CAD build for the part. Positions are in the model's coordinates, mm. A direction names the side the tool comes from. Coordinates: 2 decimals unless noted, no trailing zeros. Loops run counter-clockwise (first coordinate to the right, second up) from the corner with the lowest first, then second, coordinate; pieces in that order, holes last.
1) Two-plate mould, pull along X, no slides. Class faces 1 (the flat face through (-20, 3, -15)), 2 (the flat face through (-33.8, 5, -23)), 3 (the flat face through (-53, 3, -10)): +X half, -X half, draft (parallel to the pull), parting line (faces both ways), or undercut.
2) Pin check, flat tips, straight feed: pin 1 Ø3.5 at (x, z) = (-24.5, -27) entering from +Y; pin 2 Ø1 at (y, z) = (5, -1.5) entering from +X; pin 3 Ø5.5 at (x, z) = (-82.5, -6) entering from +Y; pin 4 Ø4 at (x, z) = (-81.5, -4.5) entering from -Y. Stop position of each tip, or through.
3) Saw through at A-A, the plane x = -59.5. Write the cut outline in (y, z), and give its area (3 significant figures).
4) Wall check: line 1 along X through (y, z) = (3.5, -13); line 2 along Z through (x, y) = (-41, 1.5); line 3 along X through (y, z) = (2.5, -6). Give the ranges that are in metal, low to high.
5) Saw through at D-D, the plane y = 5.75. Write the cut outline in (x, z).
6) Saw through at B-B, the plane z = -14.5. Write the cut outline in (x, y).
7) Saw through at C-C, the plane x = -82.5. Write the cut outline in (y, z), and give its area (3 significant figures).
8) Which spindle directions (+Z, -Z, +X, -X, +Y, -Y) get a long thin tool onto all of the face, cutting with end or side? Do faces 4 (the flat face through (-85.1, 4, -23.9)), 5 (the cylindrical face through (-38.4, 3.45, -10.57)), 6 (the flat face through (-27.8, 5, -1)). Say none if no direction does.
```python
from build123d import *

# Parameters (mm, degrees)
SKETCH_1_W           = 88
SKETCH_1_H           = 30
EXTRUDE_1_DEPTH      = 3
SKETCH_2_W           = 27.8
SKETCH_2_H           = 30
CUT_EXTRUDE_1_DEPTH  = 1
SKETCH_3_R           = 1.45
CUT_EXTRUDE_2_DEPTH  = 11
SKETCH_4_R           = 2.45
CUT_EXTRUDE_4_DEPTH  = 11
SKETCH_5_W           = 30.2
SKETCH_5_H           = 10
CUT_EXTRUDE_5_DEPTH  = 11
FILLET_1_R           = 2
SKETCH_6_W           = 5
SKETCH_6_H           = 30
CUT_EXTRUDE_6_DEPTH  = 10
SKETCH_9_W           = 60.2
SKETCH_9_H           = 30
SKETCH_9_R           = 2.45
EXTRUDE_4_DEPTH      = 4
EXTRUDE_START        = 1
SKETCH_7_W           = 22.8
SKETCH_7_H           = 30
SKETCH_7_R           = 1.45
EXTRUDE_5_DEPTH      = 1
SKETCH_11_W          = 15
SKETCH_11_H          = 4
CUT_EXTRUDE_8_DEPTH  = 6
SKETCH_12_W          = 2
SKETCH_12_H          = 4
EXTRUDE_6_DEPTH      = 6
SKETCH_13_W          = 6
SKETCH_13_H          = 4
EXTRUDE_7_DEPTH      = 4
SKETCH_14_R          = 4
CUT_EXTRUDE_9_DEPTH  = 4
SKETCH_15_W          = 9
SKETCH_15_H          = 4
CUT_EXTRUDE_10_DEPTH = 6


with BuildPart() as part:
    # 草图1 → 凸台-拉伸1 (new body)
    with BuildSketch(Plane(origin=(0, 0, 0), x_dir=(1, 0, 0), z_dir=(0, 1, 0))):
        with Locations((-44, 15)):
            Rectangle(SKETCH_1_W, SKETCH_1_H)
    extrude(amount=EXTRUDE_1_DEPTH)

    # 草图2 → 切除-拉伸1 (cut)
    with BuildSketch(Plane(origin=(0, 3, 0), x_dir=(1, 0, 0), z_dir=(0, 1, 0))):
        with Locations((-13.9, 15)):
            Rectangle(SKETCH_2_W, SKETCH_2_H)
    extrude(amount=-CUT_EXTRUDE_1_DEPTH, mode=Mode.SUBTRACT)

    # 草图3 → 切除-拉伸2 (cut)
    with BuildSketch(Plane(origin=(0, 2, 0), x_dir=(1, 0, 0), z_dir=(0, 1, 0))):
        with Locations(Location((-24.5, 27, 0), (0, 0, 270))):
            Circle(SKETCH_3_R)
        with Locations(Location((-24.5, 3, 0), (0, 0, 270))):
            Circle(SKETCH_3_R)
        with Locations(Location((-10.5, 3, 0), (0, 0, 270))):
            Circle(SKETCH_3_R)
        with Locations(Location((-10.5, 27, 0), (0, 0, 270))):
            Circle(SKETCH_3_R)
    extrude(amount=-CUT_EXTRUDE_2_DEPTH, mode=Mode.SUBTRACT)

    # 草图4 → 切除-拉伸4 (cut)
    with BuildSketch(Plane(origin=(0, 3, 0), x_dir=(1, 0, 0), z_dir=(0, 1, 0))):
        with Locations(Location((-82.5, 24, 0), (0, 0, 270))):
            Circle(SKETCH_4_R)
        with Locations(Location((-82.5, 6, 0), (0, 0, 270))):
            Circle(SKETCH_4_R)
    extrude(amount=-CUT_EXTRUDE_4_DEPTH, mode=Mode.SUBTRACT)

    # 草图5 → 切除-拉伸5 (cut)
    with BuildSketch(Plane(origin=(0, 3, 0), x_dir=(1, 0, 0), z_dir=(0, 1, 0))):
        with Locations((-52.9, 15)):
            Rectangle(SKETCH_5_W, SKETCH_5_H)
    extrude(amount=-CUT_EXTRUDE_5_DEPTH, mode=Mode.SUBTRACT)

    # 圆角1
    fillet_1_edges = [part.edges().sort_by_distance(p)[0] for p in [
        (-68, 1.5, -10),
        (-68, 1.5, -20),
        (-37.8, 1.5, -20),
        (-37.8, 1.5, -10),
    ]]
    fillet(fillet_1_edges, radius=FILLET_1_R)

    # 草图6 → 切除-拉伸6 (cut)
    with BuildSketch(Plane.XZ):
        with Locations((-2.5, -15)):
            Rectangle(SKETCH_6_W, SKETCH_6_H)
    extrude(amount=-CUT_EXTRUDE_6_DEPTH, mode=Mode.SUBTRACT)

    # 草图9 → 凸台-拉伸4 (add)
    with BuildSketch(Plane(origin=(0, 3, 0), x_dir=(1, 0, 0), z_dir=(0, 1, 0))):
        with Locations((-57.9, 15)):
            Rectangle(SKETCH_9_W, SKETCH_9_H)
        with Locations(Location((-82.5, 6, 0), (0, 0, 270))):
            Circle(SKETCH_9_R, mode=Mode.SUBTRACT)
        with Locations(Location((-82.5, 24, 0), (0, 0, 270))):
            Circle(SKETCH_9_R, mode=Mode.SUBTRACT)
        with BuildLine():
            Line((-37.8, 12), (-37.8, 18))
            ThreePointArc((-37.8, 18), (-38.385786438, 19.414213562), (-39.8, 20))
            Line((-39.8, 20), (-66, 20))
            ThreePointArc((-66, 20), (-67.414213562, 19.414213562), (-68, 18))
            Line((-68, 18), (-68, 12))
            ThreePointArc((-68, 12), (-67.414213562, 10.585786438), (-66, 10))
            Line((-66, 10), (-39.8, 10))
            ThreePointArc((-39.8, 10), (-38.385786438, 10.585786438), (-37.8, 12))
        make_face(mode=Mode.SUBTRACT)
    extrude(amount=EXTRUDE_4_DEPTH)

    # 草图7 → 凸台-拉伸5 (add)
    with BuildSketch(Plane(origin=(0, 2, 0), x_dir=(1, 0, 0), z_dir=(0, 1, 0)).offset(EXTRUDE_START)):
        with Locations((-16.4, 15)):
            Rectangle(SKETCH_7_W, SKETCH_7_H)
        with Locations(Location((-10.5, 3, 0), (0, 0, 270))):
            Circle(SKETCH_7_R, mode=Mode.SUBTRACT)
        with Locations(Location((-24.5, 27, 0), (0, 0, 270))):
            Circle(SKETCH_7_R, mode=Mode.SUBTRACT)
        with Locations(Location((-10.5, 27, 0), (0, 0, 270))):
            Circle(SKETCH_7_R, mode=Mode.SUBTRACT)
        with Locations(Location((-24.5, 3, 0), (0, 0, 270))):
            Circle(SKETCH_7_R, mode=Mode.SUBTRACT)
    extrude(amount=-EXTRUDE_5_DEPTH)

    # 草图11 → 切除-拉伸8 (cut)
    with BuildSketch(Plane(origin=(-27.8, 0, 0), x_dir=(0, 0, -1), z_dir=(1, 0, 0))):
        with Locations((22.5, 5)):
            Rectangle(SKETCH_11_W, SKETCH_11_H)
    extrude(amount=-CUT_EXTRUDE_8_DEPTH, mode=Mode.SUBTRACT)

    # 草图12 → 凸台-拉伸6 (add)
    with BuildSketch(Plane(origin=(-33.8, 0, 0), x_dir=(0, 0, -1), z_dir=(1, 0, 0))):
        with Locations((29, 5)):
            Rectangle(SKETCH_12_W, SKETCH_12_H)
    extrude(amount=EXTRUDE_6_DEPTH)

    # 草图13 → 凸台-拉伸7 (add)
    with BuildSketch(Plane(origin=(0, 0, -15), x_dir=(-1, 0, 0), z_dir=(0, 0, -1))):
        with Locations((30.8, 5)):
            Rectangle(SKETCH_13_W, SKETCH_13_H)
    extrude(amount=EXTRUDE_7_DEPTH)

    # 草图14 → 切除-拉伸9 (cut)
    with BuildSketch(Plane.XZ):
        with Locations(Location((-82.5, -6, 0), (0, 0, 270))):
            Circle(SKETCH_14_R)
        with Locations(Location((-82.5, -24, 0), (0, 0, 270))):
            Circle(SKETCH_14_R)
    extrude(amount=-CUT_EXTRUDE_9_DEPTH, mode=Mode.SUBTRACT)

    # 草图15 → 切除-拉伸10 (cut)
    with BuildSketch(Plane(origin=(-27.8, 0, 0), x_dir=(0, 0, -1), z_dir=(1, 0, 0))):
        with Locations((6.5, 5)):
            Rectangle(SKETCH_15_W, SKETCH_15_H)
    extrude(amount=-CUT_EXTRUDE_10_DEPTH, mode=Mode.SUBTRACT)


solid = part.part
```
Data:
1. face 1: draft
1. face 2: +X half
1. face 3: undercut
2. pin 1: stops at y = 3
2. pin 2: stops at x = -27.8
2. pin 3: stops at y = 7
2. pin 4: stops at y = 4
3. outline: (0, -30) - (7, -30) - (7, -20) - (0, -20) - close; (0, -10) - (7, -10) - (7, 0) - (0, 0) - close
3. area: 140 mm2
4. line 1: x = -88 to -68, -37.8 to -27.8
4. line 2: z = -30 to -20, -10 to 0
4. line 3: x = -88 to -86.5, -78.5 to -5
5. outline: (-88, -30) - (-27.8, -30) - (-27.8, -28) - (-33.8, -28) - (-33.8, -19) - (-27.8, -19) - (-27.8, -11) - (-33.8, -11) - (-33.8, -2) - (-27.8, -2) - (-27.8, 0) - (-88, 0) - close; hole circle Ø4.9 at (-82.5, -24); hole circle Ø4.9 at (-82.5, -6); hole (-68, -18) arc R2 ccw to (-66, -20) - (-39.8, -20) arc R2 ccw to (-37.8, -18) - (-37.8, -12) arc R2 ccw to (-39.8, -10) - (-66, -10) arc R2 ccw to (-68, -12) - close
6. outline: (-88, 0) - (-68, 0) - (-68, 7) - (-88, 7) - close; (-37.8, 0) - (-5, 0) - (-5, 3) - (-27.8, 3) - (-27.8, 7) - (-37.8, 7) - close
7. outline: (0, -30) - (7, -30) - (7, -26.45) - (4, -26.45) - (4, -28) - (0, -28) - close; (0, -20) - (4, -20) - (4, -21.55) - (7, -21.55) - (7, -8.45) - (4, -8.45) - (4, -10) - (0, -10) - close; (0, -2) - (4, -2) - (4, -3.55) - (7, -3.55) - (7, 0) - (0, 0) - close
7. area: 117 mm2
8. face 4: -Y
8. face 5: +Y, -Y
8. face 6: +Z, -Z, +X, +Y
